Part model, mm, in its own coordinate system. Face numbers are marked on the shaded views. A direction names the side the tool comes from. Round coordinates to 2 decimals unless told otherwise and drop trailing zeros. Write each loop counter-clockwise with the first axis right and the second up, starting at its lowest first coordinate (ties: lowest second). Pieces come first, ordered by that corner, then holes. Notation, with made-up numbers: M 3.5,6.5 L 9.5,6.5 A16 cw 9.5,32.5 Z; hole C 78.5,31 d7. An arc over 180 degrees is marked long. Answer as a JSON object with one key per item and string values. Group by question number.
1. Drill centre lines: line 1 (X direction, y = 2.15, z = 4) (3 decimals); line 2 (X direction, y = 5.5, z = 17); line 3 (Z direction, x = 24.5, y = 14). Where is each one in solid material? Low to high. Write a range as from..to.
2. Band-saw the part on B-B, the plane y = 1.75. Write the cut outline in (x, z) (3 decimals), plus the area to 3 significant figures.
3. Band-saw the part on C-C, the plane x = 12. Write the cut outline in (y, z) (3 decimals).
4. Band-saw the part on D-D, the plane y = 7.75. Write the cut outline in (x, z).
5. Band-saw the part on A-A, the plane z = 4. Write the cut outline in (x, y) (3 decimals), plus the area to 3 significant figures.
6. Which spindle directions (+Z, -Z, +X, -X, +Y, -Y) get a long thin tool onto all of the face, cutting with end or side? Do the marked faces 1, 2, 3, 4 and 5. Say none if no direction does.
7. Drop flat-ended pins along their axis: pin 1 (2.5 mm diameter, centred on y = 2, z = 10, fed in from +X); pin 2 (2 mm diameter, centred on y = 6, z = 18, fed in from -X); pin 3 (1.5 mm diameter, centred on x = 14, y = 16.5, fed in from -Z). Give the stop position or say it passes through.
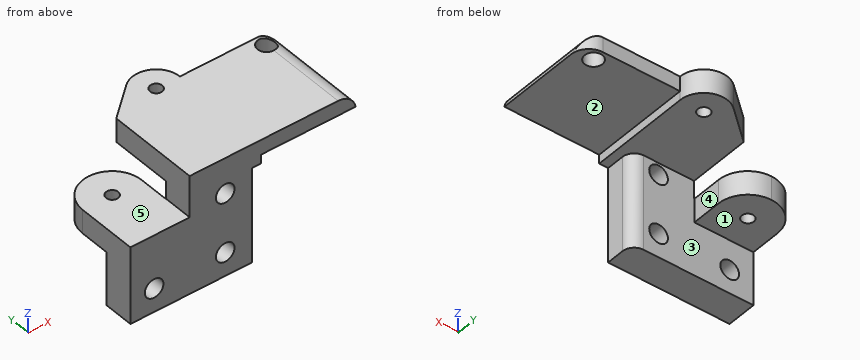
from build123d import *

# Parameters (mm, degrees)
RESSALTO_EXTRUS_O1_DEPTH                  = 20
CORTE_EXTRUS_O1_DEPTH                     = 20
CORTE_EXTRUS_O2_DEPTH                     = 34.12099032335839
RESSALTO_EXTRUS_O2_DEPTH                  = 10
FURO_ROSCADO_PARA_CONDU_TE_DE_M3X0_51_D   = 3.15
ESBO_O20_W                                = 9.95
ESBO_O20_H                                = 4.000000000000002
RESSALTO_EXTRUS_O6_DEPTH                  = 10
FILETE3_R                                 = 4.975
BROCA_DE_ROSQUEAR_PARA_TARRAXA_DE_M2_54_D = 2.05
CORTE_EXTRUS_O3_DEPTH                     = 31.199337741083
FILETE5_R                                 = 2
BROCA_DE_ROSQUEAR_PARA_TARRAXA_DE_M2_55_D = 2.05
ESBO_O30_W                                = 2.5
ESBO_O30_H                                = 17
RESSALTO_EXTRUS_O9_DEPTH                  = 16
FILETE12_R                                = 3
ESBO_O31_R                                = 1.5000000000000009
CORTE_EXTRUS_O4_DEPTH                     = 44.18564583747706


# Some blends are built 0.0001 mm under size
with BuildPart() as part:
    # Esboço1 → Ressalto-extrusão1 (new body)
    with BuildSketch(Plane.XY):
        with BuildLine():
            Line((0, 0), (0, 12))
            Line((0, 12), (9.40008084297598, 20.03980597685765))
            ThreePointArc((9.40008084297598, 20.03980597685765), (13.67336836528959, 20.633158173552044), (16, 17))
            Line((16, 17), (16, 4))
            Line((16, 4), (16, 0))
            Line((16, 0), (0, 0))
        make_face()
    extrude(amount=RESSALTO_EXTRUS_O1_DEPTH)

    # Esboço2 → Corte-extrusão1 (cut)
    with BuildSketch(Plane(origin=(16, 0, 0), x_dir=(0, 0, -1), z_dir=(1, 0, 0))):
        Polygon((0, 5), (-16, 4.999999999999997), (-16, 21), (0, 21), align=None)
    extrude(amount=-CORTE_EXTRUS_O1_DEPTH, mode=Mode.SUBTRACT)

    # Esboço3 → Corte-extrusão2 (cut, through all)
    with BuildSketch(Plane.XY.offset(20)):
        Polygon((0, 0), (4, 0), (4, 15.421164609606624), (0, 12), align=None)
    extrude(amount=-CORTE_EXTRUS_O2_DEPTH, mode=Mode.SUBTRACT)

    # Esboço8 → Ressalto-extrusão2 (add)
    with BuildSketch(Plane.ZY.offset(-4)):
        Polygon((0, 5), (13, 4.999999999999998), (13, 0), (0, 0), align=None)
    extrude(amount=RESSALTO_EXTRUS_O2_DEPTH)

    # Furo roscado para conduíte de M3x0.51 (through all)
    with Locations(Plane(origin=(-2, 0, 4), x_dir=(0, 0, -1), z_dir=(0, -1, 0))):
        with Locations((0, 0), (0, 12), (-10, 12)):
            Hole(FURO_ROSCADO_PARA_CONDU_TE_DE_M3X0_51_D / 2)

    # Esboço20 → Ressalto-extrusão6 (add)
    with BuildSketch(Plane(origin=(0, 5, 8.1e-16), x_dir=(1, 0, 0), z_dir=(0, 1, 1.6e-16))):
        with Locations((-1.025, -11)):
            Rectangle(ESBO_O20_W, ESBO_O20_H)
    extrude(amount=RESSALTO_EXTRUS_O6_DEPTH)

    # Filete3
    filete3_edges = [part.edges().sort_by_distance(p)[0] for p in [
        (3.95, 14.999999999999998, 11.000000000000002),
        (-6, 14.999999999999998, 11.000000000000002),
    ]]
    fillet(filete3_edges, radius=FILETE3_R - 0.0001)  # a hair under: the kernel refuses the full size

    # Broca de rosquear para tarraxa de M2.54 (through all)
    with Locations(Plane.XY.offset(13)):
        with Locations((-1.025, 10.025)):
            Hole(BROCA_DE_ROSQUEAR_PARA_TARRAXA_DE_M2_54_D / 2)

    # Esboço24 → Corte-extrusão3 (cut, through all)
    with BuildSketch(Plane(origin=(0, 5, 8.1e-16), x_dir=(1, 0, 0), z_dir=(0, 1, 1.6e-16))):
        Polygon((16, 8.1e-16), (14.5, -1.8e-16), (14.500000000000002, -15.999999999999996), (16, -15.999999999999996), align=None)
    extrude(amount=-CORTE_EXTRUS_O3_DEPTH, mode=Mode.SUBTRACT)

    # Filete5
    filete5_edges = [part.edges().sort_by_distance(p)[0] for p in [
        (14.5, 4.999999999999999, 7.999999999999999),
    ]]
    fillet(filete5_edges, radius=FILETE5_R)

    # Broca de rosquear para tarraxa de M2.55 (through all)
    with Locations(Plane.XY.offset(20)):
        with Locations((12, 17)):
            Hole(BROCA_DE_ROSQUEAR_PARA_TARRAXA_DE_M2_55_D / 2)

    # Esboço30 → Ressalto-extrusão9 (add)
    with BuildSketch(Plane(origin=(16, 0, 0), x_dir=(0, 0, -1), z_dir=(1, 0, 0))):
        with Locations((-18.75, 8.5)):
            Rectangle(ESBO_O30_W, ESBO_O30_H)
    extrude(amount=RESSALTO_EXTRUS_O9_DEPTH)

    # Filete12
    # the kernel refuses this fillet: 3 mm, written as the material it takes off along each edge
    with BuildSketch(Plane(origin=(32, 17, 10), x_dir=(-1, 0, 0), z_dir=(0, 0, 1))) as filete12_piece_1:
        with BuildLine():
            CenterArc((FILETE12_R, FILETE12_R), FILETE12_R, 180, 90)
            Line((0, FILETE12_R), (-FILETE12_R * 0.02, FILETE12_R))
            Line((-FILETE12_R * 0.02, FILETE12_R), (-FILETE12_R * 0.02, -FILETE12_R * 0.02))
            Line((-FILETE12_R * 0.02, -FILETE12_R * 0.02), (FILETE12_R, -FILETE12_R * 0.02))
            Line((FILETE12_R, -FILETE12_R * 0.02), (FILETE12_R, 0))
        make_face()
    extrude(amount=17.5, mode=Mode.SUBTRACT)
    with BuildSketch(Plane(origin=(32, 24.39509972887527, 20), x_dir=(-1.1653e-13, 0, -1), z_dir=(0, -1, 0))) as filete12_piece_2:
        with BuildLine():
            CenterArc((3.0000000000003446, -2.9580398915497583), FILETE12_R, 99.59406822686617, 80.40593177314054)
            Line((3.447e-13, -2.958039891550108), (-0.05999999999965402, -2.958039891550115))
            Line((-0.05999999999965402, -2.958039891550115), (-0.05999999999999872, -6.99e-15))
            Line((-0.05999999999999872, -6.99e-15), (-6.99e-15, 0.06000000000000227))
            ThreePointArc((-6.99e-15, 0.06000000000000227), (1.250000000000018, 0.06000000000014793), (2.4900000000000446, 0.05916079783099687))
            Line((2.4900000000000446, 0.05916079783099687), (2.5000000000000497, 0))
        make_face()
    extrude(amount=31.79019945775054, mode=Mode.SUBTRACT)

    # Esboço31 → Corte-extrusão4 (cut, through all)
    with BuildSketch(Plane.XY.offset(20)):
        with Locations((29, 15.000000000000002)):
            Circle(ESBO_O31_R)
    extrude(amount=-CORTE_EXTRUS_O4_DEPTH, mode=Mode.SUBTRACT)


solid = part.part
Worked answers:
{
 "1": {"line 1": "x = -6..-3.575, -0.425..8.425, 11.575..14.5", "line 2": "x = 4..16", "line 3": "z = 17.5..20"},
 "2": {"outline": "M -6,0 L 14.5,0 L 14.5,16 L 16,16 L 16,17.5 L 32,17.5 A3 ccw 29.042,20 L 4,20 L 4,13 L -6,13 Z; hole C -2,4 d3.15; hole C 10,4 d3.15; hole C 10,14 d3.15", "area": "361 mm^2"},
 "3": {"outline": "M 0,0 L 5,0 L 5,16 L 15.975,16 L 15.975,20 L 0,20 Z; M 18.025,16 L 21,16 L 21,20 L 18.025,20 Z"},
 "4": {"outline": "M -6,9 L 3.95,9 L 3.95,13 L -6,13 Z; M 4,16 L 16,16 L 16,17.5 L 32,17.5 A3 ccw 29.04,20 L 4,20 Z"},
 "5": {"outline": "M -6,0 L -3.575,0 L -3.575,5 L -6,5 Z; M -0.425,0 L 8.425,0 L 8.425,5 L -0.425,5 Z; M 11.575,0 L 14.5,0 L 14.5,3 A2 ccw 12.5,5 L 11.575,5 Z", "area": "70.1 mm^2"},
 "6": {"face 1": "-Z, +X, -X, +Y", "face 2": "-Z, +X, +Y, -Y", "face 3": "-Z, +X, +Y", "face 4": "+Z, -Z, +X, +Y", "face 5": "+Z, -X, +Y, -Y"},
 "7": {"pin 1": "stops at x = 14.5", "pin 2": "stops at x = 4", "pin 3": "stops at z = 16"}
}
